Part print with two shaded views. Sizes in mm from the minimum x, y, z corner. A direction names the side the tool comes from. Give positions to 0.01 mm unless a question says otherwise; leave off trailing zeros. Order: outer loops, then holes, each group sorted by start corner. A loop starts at its lowest first (then second) coordinate and runs counter-clockwise, first axis right, second up. Notation, with made-up numbers: (69.5, -38.5) -> (97.5, -38.5) arc R18 cw to (97.5, -23.5) -> close; hole circle Ø2 at (-14.5, -20.5). An arc over 180 degrees is marked (long way). Write item = value, one per line. Start each with the question number.
Item 1: Flat gauge pins, fed straight in: P1, Ø8, axis at x = 4, y = 14, coming from the -Z side; P2, Ø2, axis at y = 11.5, z = 1.5, coming from the -X side. Where does each tip first touch, or does it go through?
Item 2: Drill centre lines: line 1 along Y through (x, z) = (12, 26); line 2 along Z through (x, y) = (17, 5); line 3 along Z through (x, y) = (10.75, 17). Where is each one in solid material? Low to high.
Item 3: Tool access for the marked faces 5 and 6: list every direction of +Z, -Z, +X, -X, +Y, -Y with a clear straight run to the whole face (end or side of a thin tool).
Item 4: Band-saw the part on C-C on y = 3. Write the cut outline in (x, z), plus the area to 3 significant figures.
Item 5: Band-saw the part on A-A on x = 18.25. Write the cut outline in (y, z), plus the area to 3 significant figures.
Item 6: Band-saw the part on B-B on z = 13.5. Write the cut outline in (x, y), plus the area to 4 significant figures.
Item 7: Pull direction Z, two halves, no side cores. Call the marked faces 1, 2, 3 and 4: +Z half, -Z half, draft (parallel to the pull), parting line (faces both ways), or undercut.
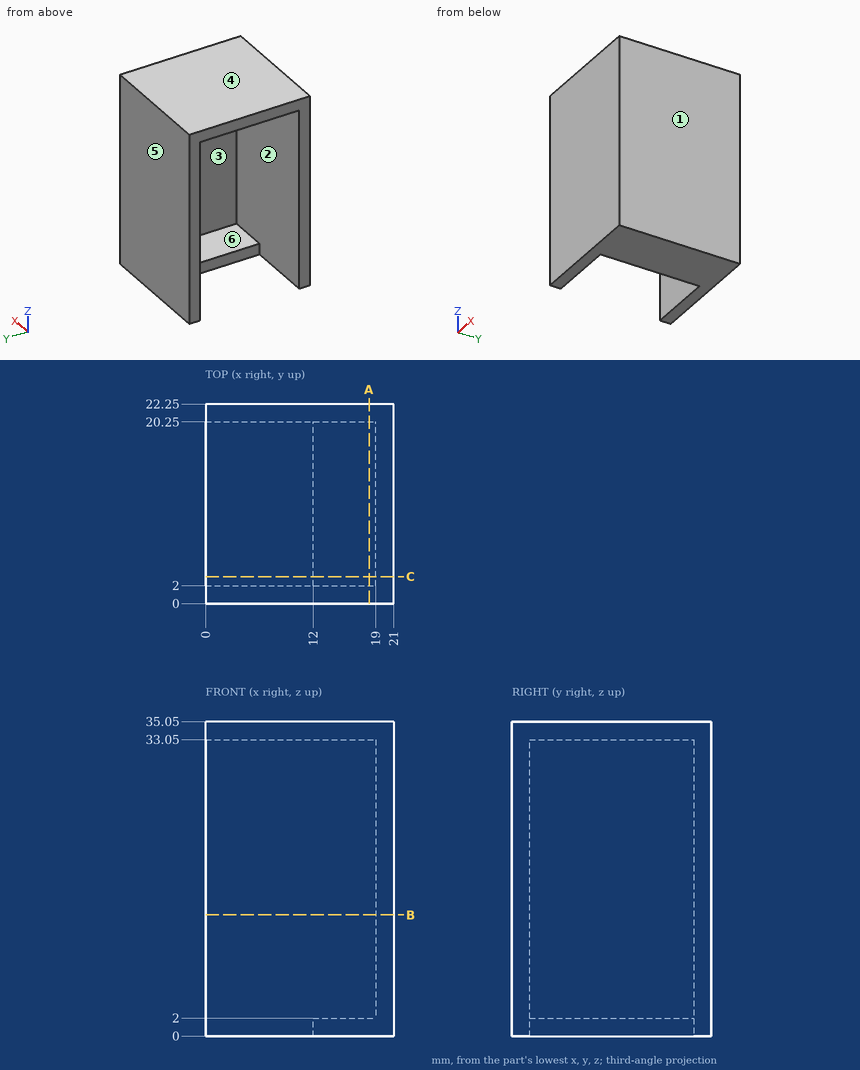
Values found:
q1.P1 = 33.05
q1.P2 = 12
q2.line_1 = 0 to 2, 20.25 to 22.25
q2.line_2 = 0 to 2, 33.05 to 35.05
q2.line_3 = 33.05 to 35.05
q3.face_5 = +Z, -Z, +X, -X, +Y
q3.face_6 = -X
q4.outline = (0, 33.05) -> (19, 33.05) -> (19, 2) -> (12, 2) -> (12, 0) -> (21, 0) -> (21, 35.05) -> (0, 35.05) -> close
q4.area = 122 mm^2
q5.outline = (0, 0) -> (22.25, 0) -> (22.25, 35.05) -> (0, 35.05) -> close; hole (2, 2) -> (20.25, 2) -> (20.25, 33.05) -> (2, 33.05) -> close
q5.area = 213 mm^2
q6.outline = (0, 0) -> (21, 0) -> (21, 22.25) -> (0, 22.25) -> (0, 20.25) -> (19, 20.25) -> (19, 2) -> (0, 2) -> close
q6.area = 120.5 mm^2
q7.face_1 = draft
q7.face_2 = undercut
q7.face_3 = undercut
q7.face_4 = +Z half
